Build history of the part. All positions in model axes, mm. Give positions to 0.01 mm unless a question says otherwise; leave off trailing zeros. Loops run counter-clockwise (first coordinate to the right, second up) from the corner with the lowest first, then second, coordinate; pieces in that order, holes last. Notation, with made-up numbers: (80.25, 36) -> (117.25, 36) arc R20 ccw to (117.25, 65) -> close; hole circle Ø3 at (-15, 57). An arc over 180 degrees is marked (long way). Answer in a Markdown table with one row per item. Add a question column.
from build123d import *

# Parameters (mm, degrees)
SKETCH6_R                = 241.3
SKETCH6_R_2              = 190.5
BOSS_EXTRUDE1_DEPTH      = 12.7
F_7_8_1_DIAMETER_HOLE1_D = 25.4
CIRPATTERN1_COUNT        = 12


with BuildPart() as part:
    # Sketch6 → Boss-Extrude1 (new body, symmetric)
    with BuildSketch(Plane(origin=(0, 0, 0), x_dir=(0, 0, -1), z_dir=(1, 0, 0))):
        with Locations((0, 316.3)):
            Circle(SKETCH6_R)
        with Locations((0, 316.3)):
            Circle(SKETCH6_R_2, mode=Mode.SUBTRACT)
    extrude(amount=BOSS_EXTRUDE1_DEPTH, both=True)

    # 7_8 _1_ Diameter Hole1 (through all)
    with Locations(Plane(origin=(12.7, 0, 0), x_dir=(0, 0, -1), z_dir=(1, 0, 0))):
        with Locations((208.543385896, 260.420968162)):
            f_7_8_1_diameter_hole1 = Hole(F_7_8_1_DIAMETER_HOLE1_D / 2)

    # CirPattern1: 7_8 _1_ Diameter Hole1 ×12 about axis
    cirpattern1_axis = Axis((0, 316.3, 0), (1, 0, 0))
    for i in range(1, CIRPATTERN1_COUNT):
        add(f_7_8_1_diameter_hole1.rotate(cirpattern1_axis, i * 360 / CIRPATTERN1_COUNT), mode=Mode.SUBTRACT)


solid = part.part
(1) Flat gauge pins, fed straight in: pin 1 Ø4 at (x, z) = (0.5, 65.5) entering from +Y; pin 2 Ø6 at (x, z) = (-10, -132.5) entering from +Y; pin 3 Ø5 at (x, y) = (6.5, 124.5) entering from -Z. Where does each tip first touch, or does it go through?
(2) Two-plate mould, pull along Z, no slides. Class faces 1 (the cylindrical face through (-0.178, 537.435, 54.226)), 2 (the cylindrical face through (0.18, 80.74, 52.31)), 3 (the flat face through (-12.7, 389, -178)): released by +Z, released by -Z, zero draft, split by the parting line, or undercut.
(3) Saw through at A-A, the plane z = 0. List the corners of the cut face in (x, y).
(4) Wall check: line 1 along Y through (x, z) = (-10.25, 61); line 2 along Y through (x, z) = (-0.75, -48); line 3 along Z through (x, y) = (3.75, 168). Give the ranges that are in metal, low to high. Write a range as from..to.
(5) Saw through at D-D, the plane y = 109.5. List the corners of the cut face in (x, z).
(6) Saw through at C-C, the plane x = 7. State how many separate pieces and enclosed holes the cut face has, then the cut area to 3 significant figures.
(7) Saw through at B-B, the plane y = 316.3. List the corners of the cut face in (x, z).
Worked answers:
| question | item | result |
|---|---|---|
| 1 | pin 1 | y = 549.09 |
| 1 | pin 2 | y = 519.91 |
| 1 | pin 3 | z = -149.64 |
| 2 | face 1 | undercut |
| 2 | face 2 | split by the parting line |
| 2 | face 3 | zero draft |
| 3 | outline | (-12.7, 75) -> (12.7, 75) -> (12.7, 125.8) -> (-12.7, 125.8) -> close; (-12.7, 506.8) -> (12.7, 506.8) -> (12.7, 557.6) -> (-12.7, 557.6) -> close |
| 4 | line 1 | 82.84..96.13, 119.38..135.83, 496.77..513.22, 536.47..549.76 |
| 4 | line 2 | 79.82..97.8, 117.72..131.95, 500.65..514.88, 534.8..552.78 |
| 4 | line 3 | -190.35..-164.59, -140.74..-119.57, 119.57..140.74, 164.59..190.35 |
| 5 | outline | (-12.7, -124.34) -> (12.7, -124.34) -> (12.7, -68.46) -> (-12.7, -68.46) -> close; (-12.7, -43.3) -> (12.7, -43.3) -> (12.7, 43.3) -> (-12.7, 43.3) -> close; (-12.7, 68.46) -> (12.7, 68.46) -> (12.7, 124.34) -> (-12.7, 124.34) -> close |
| 6 | separate pieces | 1 |
| 6 | enclosed holes | 13 |
| 6 | area | 62,800 mm^2 |
| 7 | outline | (-12.7, -241.3) -> (12.7, -241.3) -> (12.7, -190.5) -> (-12.7, -190.5) -> close; (-12.7, 190.5) -> (12.7, 190.5) -> (12.7, 241.3) -> (-12.7, 241.3) -> close |
